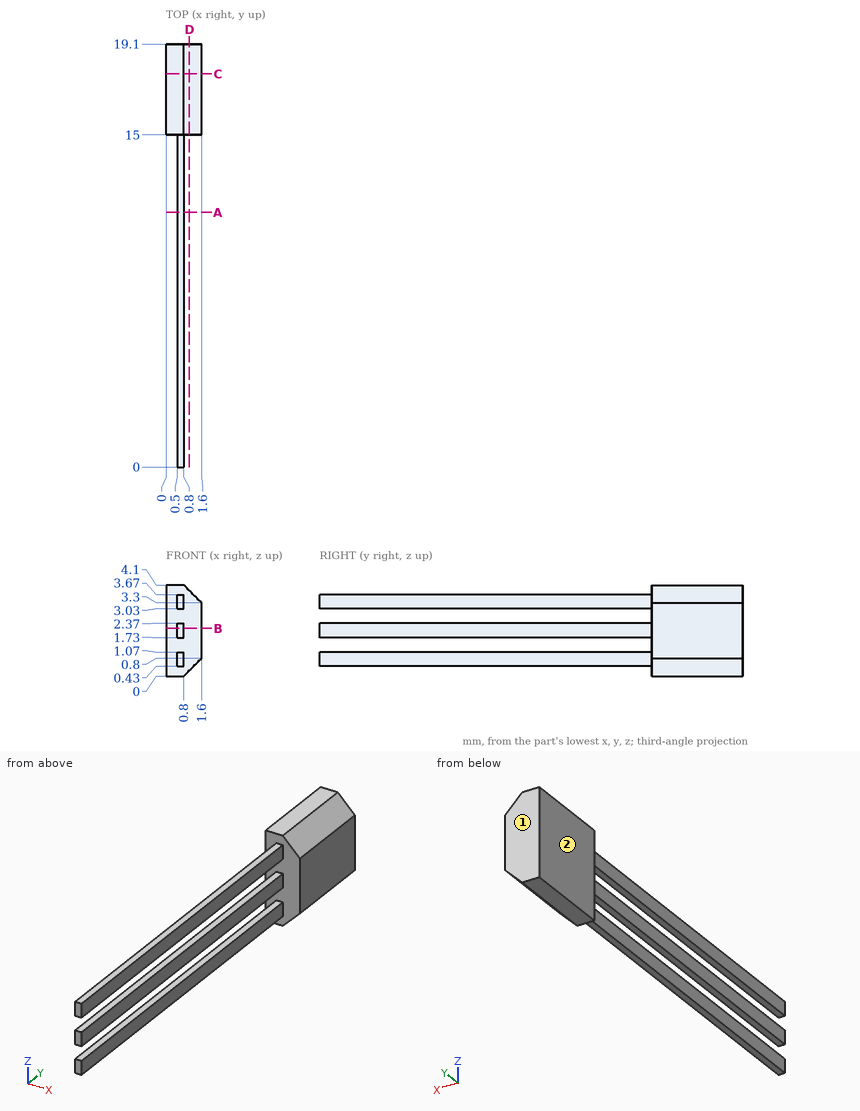
Geometry check sheet. Reference: drawing and pictorial views, mm from the part's lowest x, y, z. Round coordinates to 2 decimals unless told otherwise and drop trailing zeros. Order: outer loops, then holes, each group sorted by start corner. A loop starts at its lowest first (then second) coordinate and runs counter-clockwise, first axis right, second up. Notation, with made-up numbers: M -37.75,48 L -22.75,48 A11 cw -22.75,64 Z; hole C 55,19.25 d7. An arc over 180 degrees is marked long. Write item = value, one per line.
Q1. Section check A-A (y = 11.5). Enter the section's corners in (x, z), plus the area to 3 significant figures.
Answer block:
outline = M 0.5,0.43 L 0.8,0.43 L 0.8,1.07 L 0.5,1.07 Z; M 0.5,1.73 L 0.8,1.73 L 0.8,2.37 L 0.5,2.37 Z; M 0.5,3.03 L 0.8,3.03 L 0.8,3.67 L 0.5,3.67 Z
area = 0.576 mm^2
Q2. Section check B-B (z = 2.15). Enter the section's corners in (x, y), plus the area to 3 significant figures.
Answer block:
outline = M 0,15 L 0.5,15 L 0.5,0 L 0.8,0 L 0.8,15 L 1.6,15 L 1.6,19.1 L 0,19.1 Z
area = 11.1 mm^2
Q3. Depth check by flat-ended pin: pin 1 Ø0.7 at (y, z) = (7, 2) entering from +X; pin 2 Ø0.5 at (y, z) = (7, 2) entering from -X. Enter the tip coordinate at first touch or a pass-through.
Answer block:
pin_1 = 0.8
pin_2 = 0.5
Q4. Section check D-D (x = 1.05). Enter the section's corners in (y, z).
Answer block:
outline = M 15,0.25 L 19.1,0.25 L 19.1,3.85 L 15,3.85 Z
Q5. Scan lines: line 1 (Z direction, x = 0.75, y = 11.5); line 2 (X direction, y = 14, z = 3.4); line 3 (Y direction, x = 1, z = 2.9). Record each from-to range of solid material in increasing order.
Answer block:
line_1 = 0.43 to 1.07, 1.73 to 2.37, 3.03 to 3.67
line_2 = 0.5 to 0.8
line_3 = 15 to 19.1
Q6. Section check C-C (y = 17.75). Enter the section's corners in (x, z).
Answer block:
outline = M 0,0 L 0.8,0 L 1.6,0.8 L 1.6,3.3 L 0.8,4.1 L 0,4.1 Z
Q7. Release check for a two-part mould opening along Y. For the marked faces 1 and 2 record: released by +Y, released by -Y, zero draft, split by the parting line, or undercut.
Answer block:
face_1 = released by +Y
face_2 = zero draft
